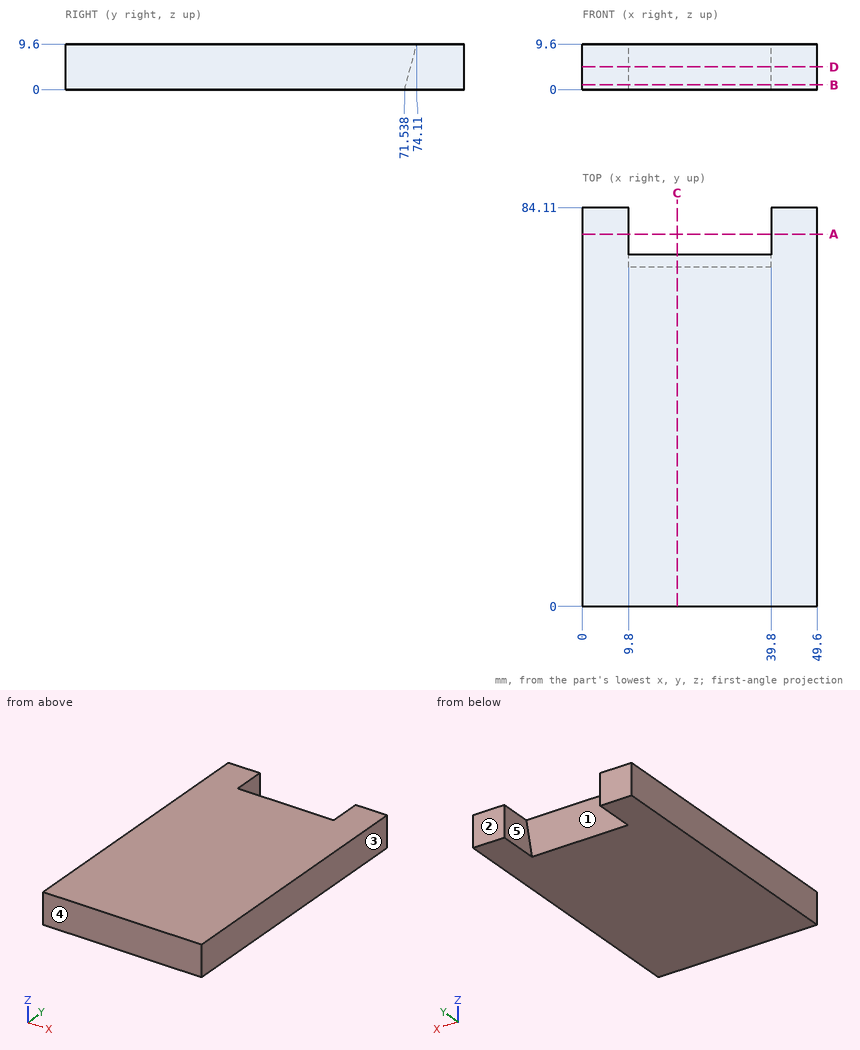
Geometry: see drawing. Coordinates: mm, zero at the bounding-box minimum. A direction names the side the tool comes from. Give positions to 0.01 mm unless a question says otherwise; leave off trailing zeros. Write each loop counter-clockwise with the first axis right and the second up, starting at its lowest first coordinate (ties: lowest second). Pieces come first, ordered by that corner, then holes. Notation, with made-up numbers: (69.25, 10) -> (97.25, 10) arc R14 cw to (97.25, 28) -> close; hole circle Ø5 at (13.25, -19.75). An arc over 180 degrees is marked (long way). Use one line per item in the form item = value. Start each with the question number.
1) Draft query along X for the marked faces 3, 4 and 5. Return one class per face: pulls with the +X half, pulls with the -X half, needs draft (parallel to the pull), parting line crosses it, or undercut.
2) Ray query, probe 1 along X at (y, z) = (76.5, 2.5); probe 2 along Y at (x, z) = (28.5, 3.5) (1 decimal); probe 3 along Y at (x, z) = (19, 9.25). Return the intervals inside material, ascending. Write a range as from..to.
3) Section query B-B on z = 1. Return the cut outline in (x, y), then the cut area to 3 significant figures.
4) Set-up query: the marked faces 1 and 2. Return all of +Z, -Z, +X, -X, +Y, -Y with unobstructed straight access to the full face (end or side cutting, diameter ignored); none if empty.
5) Section query C-C on x = 20. Return the cut outline in (y, z), then the cut area to 3 significant figures.
6) Pin query (flat end, axial travel): pin 1 (1 mm diameter, centred on x = 24.5, y = 23.5, fed in from -Z). Return the tip coordinate at first contact, or that it passes through.
7) Section query D-D on z = 4.75. Return the cut outline in (x, y).
8) Section query A-A on y = 78.5. Return the cut outline in (x, z), then the cut area to 3 significant figures.
Outcome:
q1.face_3 = pulls with the +X half
q1.face_4 = needs draft
q1.face_5 = undercut
q2.probe_1 = 0..9.8, 39.8..49.6
q2.probe_2 = 0..72.5
q2.probe_3 = 0..74.02
q3.outline = (0, 0) -> (49.6, 0) -> (49.6, 84.11) -> (39.8, 84.11) -> (39.8, 71.81) -> (9.8, 71.81) -> (9.8, 84.11) -> (0, 84.11) -> close
q3.area = 3,800 mm^2
q4.face_1 = -Z, +Y
q4.face_2 = +Z, -Z, +X, -X, +Y
q5.outline = (0, 0) -> (71.54, 0) -> (74.11, 9.6) -> (0, 9.6) -> close
q5.area = 699 mm^2
q6.pin_1 = 0
q7.outline = (0, 0) -> (49.6, 0) -> (49.6, 84.11) -> (39.8, 84.11) -> (39.8, 72.81) -> (9.8, 72.81) -> (9.8, 84.11) -> (0, 84.11) -> close
q8.outline = (0, 0) -> (9.8, 0) -> (9.8, 9.6) -> (0, 9.6) -> close; (39.8, 0) -> (49.6, 0) -> (49.6, 9.6) -> (39.8, 9.6) -> close
q8.area = 188 mm^2
